```python
from build123d import *

# Parameters (mm, degrees)
BOSS_EXTRUDE1_DEPTH = 6.1
CUT_EXTRUDE1_REACH  = 8.1
SKETCH2_R           = 0.7
CHAMFER1_SIZE       = 0.25


with BuildPart() as part:
    # Sketch1 → Boss-Extrude1 (new body)
    with BuildSketch(Plane.XY):
        with BuildLine():
            Line((-5.357339767, -3.25), (5.357339767, -3.25))
            ThreePointArc((5.357339767, -3.25), (5.813910839, -3.095015005), (6.081784137, -2.694114284))
            Line((6.081784137, -2.694114284), (7.421530099, 2.305885716))
            ThreePointArc((7.421530099, 2.305885716), (7.292100735, 2.956571072), (6.697085729, 3.25))
            Line((6.697085729, 3.25), (-6.697085729, 3.25))
            ThreePointArc((-6.697085729, 3.25), (-7.292100735, 2.956571072), (-7.421530099, 2.305885716))
            Line((-7.421530099, 2.305885716), (-6.081784137, -2.694114284))
            ThreePointArc((-6.081784137, -2.694114284), (-5.813910839, -3.095015005), (-5.357339767, -3.25))
        make_face()
    extrude(amount=BOSS_EXTRUDE1_DEPTH)

    # Sketch2 → Cut-Extrude1 (cut, up to next)
    with BuildSketch(Plane.XY.offset(6.1), mode=Mode.PRIVATE) as cut_extrude1_sk1:
        with Locations((-5.999496922, 1.5)):
            Circle(SKETCH2_R)
    cut_extrude1_tool1 = extrude(cut_extrude1_sk1.sketch, amount=-CUT_EXTRUDE1_REACH, mode=Mode.PRIVATE) & part.part
    add(cut_extrude1_tool1.solids().sort_by_distance((-5.999497, 1.5, 6.1))[0], mode=Mode.SUBTRACT)
    # Sketch2 → Cut-Extrude1 (cut, up to next)
    with BuildSketch(Plane.XY.offset(6.1), mode=Mode.PRIVATE) as cut_extrude1_sk2:
        with Locations((-2.999496922, 1.5)):
            Circle(SKETCH2_R)
    cut_extrude1_tool2 = extrude(cut_extrude1_sk2.sketch, amount=-CUT_EXTRUDE1_REACH, mode=Mode.PRIVATE) & part.part
    add(cut_extrude1_tool2.solids().sort_by_distance((-2.999497, 1.5, 6.1))[0], mode=Mode.SUBTRACT)
    # Sketch2 → Cut-Extrude1 (cut, up to next)
    with BuildSketch(Plane.XY.offset(6.1), mode=Mode.PRIVATE) as cut_extrude1_sk3:
        with Locations((0.000503078, 1.5)):
            Circle(SKETCH2_R)
    cut_extrude1_tool3 = extrude(cut_extrude1_sk3.sketch, amount=-CUT_EXTRUDE1_REACH, mode=Mode.PRIVATE) & part.part
    add(cut_extrude1_tool3.solids().sort_by_distance((0.000503, 1.5, 6.1))[0], mode=Mode.SUBTRACT)
    # Sketch2 → Cut-Extrude1 (cut, up to next)
    with BuildSketch(Plane.XY.offset(6.1), mode=Mode.PRIVATE) as cut_extrude1_sk4:
        with Locations((3.000503078, 1.5)):
            Circle(SKETCH2_R)
    cut_extrude1_tool4 = extrude(cut_extrude1_sk4.sketch, amount=-CUT_EXTRUDE1_REACH, mode=Mode.PRIVATE) & part.part
    add(cut_extrude1_tool4.solids().sort_by_distance((3.000503, 1.5, 6.1))[0], mode=Mode.SUBTRACT)
    # Sketch2 → Cut-Extrude1 (cut, up to next)
    with BuildSketch(Plane.XY.offset(6.1), mode=Mode.PRIVATE) as cut_extrude1_sk5:
        with Locations((6.000503078, 1.5)):
            Circle(SKETCH2_R)
    cut_extrude1_tool5 = extrude(cut_extrude1_sk5.sketch, amount=-CUT_EXTRUDE1_REACH, mode=Mode.PRIVATE) & part.part
    add(cut_extrude1_tool5.solids().sort_by_distance((6.000503, 1.5, 6.1))[0], mode=Mode.SUBTRACT)
    # Sketch2 → Cut-Extrude1 (cut, up to next)
    with BuildSketch(Plane.XY.offset(6.1), mode=Mode.PRIVATE) as cut_extrude1_sk6:
        with Locations((-4.499496922, -1.5)):
            Circle(SKETCH2_R)
    cut_extrude1_tool6 = extrude(cut_extrude1_sk6.sketch, amount=-CUT_EXTRUDE1_REACH, mode=Mode.PRIVATE) & part.part
    add(cut_extrude1_tool6.solids().sort_by_distance((-4.499497, -1.5, 6.1))[0], mode=Mode.SUBTRACT)
    # Sketch2 → Cut-Extrude1 (cut, up to next)
    with BuildSketch(Plane.XY.offset(6.1), mode=Mode.PRIVATE) as cut_extrude1_sk7:
        with Locations((-1.499496922, -1.5)):
            Circle(SKETCH2_R)
    cut_extrude1_tool7 = extrude(cut_extrude1_sk7.sketch, amount=-CUT_EXTRUDE1_REACH, mode=Mode.PRIVATE) & part.part
    add(cut_extrude1_tool7.solids().sort_by_distance((-1.499497, -1.5, 6.1))[0], mode=Mode.SUBTRACT)
    # Sketch2 → Cut-Extrude1 (cut, up to next)
    with BuildSketch(Plane.XY.offset(6.1), mode=Mode.PRIVATE) as cut_extrude1_sk8:
        with Locations((1.500503078, -1.5)):
            Circle(SKETCH2_R)
    cut_extrude1_tool8 = extrude(cut_extrude1_sk8.sketch, amount=-CUT_EXTRUDE1_REACH, mode=Mode.PRIVATE) & part.part
    add(cut_extrude1_tool8.solids().sort_by_distance((1.500503, -1.5, 6.1))[0], mode=Mode.SUBTRACT)
    # Sketch2 → Cut-Extrude1 (cut, up to next)
    with BuildSketch(Plane.XY.offset(6.1), mode=Mode.PRIVATE) as cut_extrude1_sk9:
        with Locations((4.500503078, -1.5)):
            Circle(SKETCH2_R)
    cut_extrude1_tool9 = extrude(cut_extrude1_sk9.sketch, amount=-CUT_EXTRUDE1_REACH, mode=Mode.PRIVATE) & part.part
    add(cut_extrude1_tool9.solids().sort_by_distance((4.500503, -1.5, 6.1))[0], mode=Mode.SUBTRACT)

    # Chamfer1
    chamfer1_edges = [part.edges().sort_by_distance(p)[0] for p in [
        (-6.699496922, 1.5, 6.1),
        (-3.699496922, 1.5, 6.1),
        (-0.699496922, 1.5, 6.1),
        (2.300503078, 1.5, 6.1),
        (5.300503078, 1.5, 6.1),
        (-5.199496922, -1.5, 6.1),
        (-2.199496922, -1.5, 6.1),
        (0.800503078, -1.5, 6.1),
        (3.800503078, -1.5, 6.1),
    ]]
    chamfer(chamfer1_edges, length=CHAMFER1_SIZE)


solid = part.part
```
For this review, take the finished solid that the model builds, in its own axes (mm). Round coordinates to 2 decimals unless told otherwise and drop trailing zeros. Loops run counter-clockwise (first coordinate to the right, second up) from the corner with the lowest first, then second, coordinate; pieces in that order, holes last.
Q1. Add section A-A on z = 5.5. Give the number of separate pieces and of enclosed holes in the cut face, plus the area to 3 significant figures.
Result sheet:
separate pieces: 1
enclosed holes: 9
area: 74.0 mm2
Q2. Add section B-B on y = -1.5. Write out the cut boundary in (x, z).
Result sheet:
outline: (-6.4, 0) - (-5.2, 0) - (-5.2, 5.85) - (-5.45, 6.1) - (-6.4, 6.1) - close; (-3.8, 0) - (-2.2, 0) - (-2.2, 5.85) - (-2.45, 6.1) - (-3.55, 6.1) - (-3.8, 5.85) - close; (-0.8, 0) - (0.8, 0) - (0.8, 5.85) - (0.55, 6.1) - (-0.55, 6.1) - (-0.8, 5.85) - close; (2.2, 0) - (3.8, 0) - (3.8, 5.85) - (3.55, 6.1) - (2.45, 6.1) - (2.2, 5.85) - close; (5.2, 0) - (6.4, 0) - (6.4, 6.1) - (5.45, 6.1) - (5.2, 5.85) - close
Q3. Insertion check: pin 1 Ø1.6 at (x, y) = (3, 1.5) entering from +Z; pin 2 Ø1.8 at (x, y) = (-3, 1.5) entering from +Z; pin 3 Ø1 at (y, z) = (1, 1.5) entering from +X. Each pin has a flat end and moves straight along its axis. Give the tip position at first contact, or say it passes through.
Result sheet:
pin 1: stops at z = 5.95
pin 2: stops at z = 6.05
pin 3: stops at x = 7.21
Q4. To check wall thickness, follow line 1 along Y through (x, z) = (-4.5, 3.25); line 2 along X through (y, z) = (-2, 4); line 3 along X through (y, z) = (1.25, 5.5). State the ranges of each line that lie inside material, in increasing order.
Result sheet:
line 1: y = -3.25 to -2.2, -0.8 to 3.25
line 2: x = -6.27 to -4.99, -4.01 to -1.99, -1.01 to 1.01, 1.99 to 4.01, 4.99 to 6.27
line 3: x = -7.14 to -6.65, -5.35 to -3.65, -2.35 to -0.65, 0.65 to 2.35, 3.65 to 5.35, 6.65 to 7.14
Q5. Mouldability with a two-part tool opening along Y and no side actions: class faces 1 (the face through (0, 0, 6.1)), 2 (the face through (0, 3.25, 3)), 3 (the face through (6.74, -0.23, 3.01)), 4 (the face through (-3.151, 0.817, 2.966)) as +Y half, -Y half, draft (parallel to the pull), parting line (faces both ways), or undercut.
Result sheet:
face 1: draft
face 2: +Y half
face 3: -Y half
face 4: undercut
